Part model, mm, in its own coordinate system. A direction names the side the tool comes from. Round coordinates to 2 decimals unless told otherwise and drop trailing zeros. Write each loop counter-clockwise with the first axis right and the second up, starting at its lowest first coordinate (ties: lowest second). Pieces come first, ordered by that corner, then holes.
1) Flat gauge pins, fed straight in: pin 1 (9.5 mm diameter, centred on x = 35, y = 222, fed in from +Z); pin 2 (1 mm diameter, centred on x = -39, z = 9.5, fed in from -Y); pin 3 (6.5 mm diameter, centred on x = -8, z = 12.5, fed in from +Y); pin 4 (6 mm diameter, centred on y = 134.5, z = 13.5, fed in from +X). Where does each tip first touch, or does it go through?
2) Drill centre lines: L1, parallel to X at y = -141, z = 15.5; L2, parallel to Y at x = 35, z = 4; L3, parallel to Y at x = 132, z = 9.5. Where is each one in solid material? Low to high.
3) Pull direction Y, two halves, no side cores. Call faces 1 (the cylindrical face through (-186.88, -102.57, 8.11)), 2 (the flat face through (-224.978, 132.327, 12.056)), 3 (the flat face through (-227.09, -128.67, 12.06)): +Y half, -Y half, draft (parallel to the pull), parting line (faces both ways), or undercut.
4) Saw through at A-A on y = -111. Write the cut outline in (x, z).
5) Saw through at C-C on x = 101.5. Write the cut outline in (y, z), and give its area (3 significant figures).
6) Which spindle directions (+Z, -Z, +X, -X, +Y, -Y) get a long thin tool onto all of the face, cutting with end or side? Do faces 4 (the flat face through (224.978, -132.327, 12.056)), 5 (the flat face through (233.598, 137.397, 3.944)), 6 (the flat face through (227.09, 128.67, 12.06)), 7 (the flat face through (-1, 262, 8)). Say none if no direction does.
7) Saw through at B-B on z = 3. Count the separate pieces of the cut face and the enclosed holes in it, and give its area (3 significant figures).
8) Saw through at D-D on y = 68.5. Write the cut outline in (x, z), and give its area (3 significant figures).
```python
from build123d import *

# Parameters (mm, degrees)
BOSS_EXTRUDE1_DEPTH = 16
CUT_EXTRUDE1_REACH  = 426.953
SKETCH3_R           = 6
SKETCH4_OUTSIDE_W   = 813.904
SKETCH4_OUTSIDE_H   = 727.89
CUT_EXTRUDE2_DEPTH  = 8
SKETCH5_R           = 1.25
SKETCH5_R_2         = 10
CUT_EXTRUDE3_DEPTH  = 425.953330771
CUT_EXTRUDE6_DEPTH  = 425.953330771


with BuildPart() as part:
    # Sketch1 → Boss-Extrude1 (new body)
    with BuildSketch(Plane.XY):
        Polygon((160.503374835, 278), (-160.503374835, 278), (-321.006749669, 0), (-160.503374835, -278), (160.503374835, -278), (321.006749669, 0), align=None)
    extrude(amount=BOSS_EXTRUDE1_DEPTH)

    # Sketch3 → Cut-Extrude1 (cut, up to next)
    with BuildSketch(Plane.XY.offset(16), mode=Mode.PRIVATE) as cut_extrude1_sk1:
        with Locations((35, 222)):
            Circle(SKETCH3_R)
    cut_extrude1_tool1 = extrude(cut_extrude1_sk1.sketch, amount=-CUT_EXTRUDE1_REACH, mode=Mode.PRIVATE) & part.part
    # Sketch3 → Cut-Extrude1 (cut, up to next)
    with BuildSketch(Plane.XY.offset(16), mode=Mode.PRIVATE) as cut_extrude1_sk2:
        with Locations((-35, 222)):
            Circle(SKETCH3_R)
    cut_extrude1_tool2 = extrude(cut_extrude1_sk2.sketch, amount=-CUT_EXTRUDE1_REACH, mode=Mode.PRIVATE) & part.part
    # Sketch3 → Cut-Extrude1 (cut, up to next)
    with BuildSketch(Plane.XY.offset(16), mode=Mode.PRIVATE) as cut_extrude1_sk3:
        with Locations((-209.75763964, -80.689110868)):
            Circle(SKETCH3_R)
    cut_extrude1_tool3 = extrude(cut_extrude1_sk3.sketch, amount=-CUT_EXTRUDE1_REACH, mode=Mode.PRIVATE) & part.part
    # Sketch3 → Cut-Extrude1 (cut, up to next)
    with BuildSketch(Plane.XY.offset(16), mode=Mode.PRIVATE) as cut_extrude1_sk4:
        with Locations((-174.75763964, -141.310889132)):
            Circle(SKETCH3_R)
    cut_extrude1_tool4 = extrude(cut_extrude1_sk4.sketch, amount=-CUT_EXTRUDE1_REACH, mode=Mode.PRIVATE) & part.part
    # Sketch3 → Cut-Extrude1 (cut, up to next)
    with BuildSketch(Plane.XY.offset(16), mode=Mode.PRIVATE) as cut_extrude1_sk5:
        with Locations((174.75763964, -141.310889132)):
            Circle(SKETCH3_R)
    cut_extrude1_tool5 = extrude(cut_extrude1_sk5.sketch, amount=-CUT_EXTRUDE1_REACH, mode=Mode.PRIVATE) & part.part
    # Sketch3 → Cut-Extrude1 (cut, up to next)
    with BuildSketch(Plane.XY.offset(16), mode=Mode.PRIVATE) as cut_extrude1_sk6:
        with Locations((209.75763964, -80.689110868)):
            Circle(SKETCH3_R)
    cut_extrude1_tool6 = extrude(cut_extrude1_sk6.sketch, amount=-CUT_EXTRUDE1_REACH, mode=Mode.PRIVATE) & part.part
    add(cut_extrude1_tool1.solids().sort_by_distance((35, 222, 16))[0], mode=Mode.SUBTRACT)
    add(cut_extrude1_tool2.solids().sort_by_distance((-35, 222, 16))[0], mode=Mode.SUBTRACT)
    add(cut_extrude1_tool3.solids().sort_by_distance((-209.75764, -80.689111, 16))[0], mode=Mode.SUBTRACT)
    add(cut_extrude1_tool4.solids().sort_by_distance((-174.75764, -141.310889, 16))[0], mode=Mode.SUBTRACT)
    add(cut_extrude1_tool5.solids().sort_by_distance((174.75764, -141.310889, 16))[0], mode=Mode.SUBTRACT)
    add(cut_extrude1_tool6.solids().sort_by_distance((209.75764, -80.689111, 16))[0], mode=Mode.SUBTRACT)

    # Sketch4 outside → Cut-Extrude2 (cut)
    with BuildSketch(Plane.XY.offset(16)):
        Rectangle(SKETCH4_OUTSIDE_W, SKETCH4_OUTSIDE_H)
        Polygon((301.376840517, 0), (150.688420258, 261), (-150.688420258, 261), (-301.376840517, 0), (-150.688420258, -261), (150.688420258, -261), align=None, mode=Mode.SUBTRACT)
    extrude(amount=-CUT_EXTRUDE2_DEPTH, mode=Mode.SUBTRACT)

    # Sketch5 → Cut-Extrude3 (cut, through all)
    with BuildSketch(Plane.XY.offset(16)):
        with Locations((209.578147716, -121)):
            Circle(SKETCH5_R)
        with Locations((174.937131564, -101)):
            Circle(SKETCH5_R)
        with Locations((-192.25763964, -111)):
            Circle(SKETCH5_R_2)
        with Locations((0, 222)):
            Circle(SKETCH5_R_2)
        with Locations((-209.578147716, -121)):
            Circle(SKETCH5_R)
        with Locations((-174.937131564, -101)):
            Circle(SKETCH5_R)
        with Locations((0, 242)):
            Circle(SKETCH5_R)
        with Locations((0, 202)):
            Circle(SKETCH5_R)
        with Locations((192.25763964, -111)):
            Circle(SKETCH5_R_2)
    extrude(amount=-CUT_EXTRUDE3_DEPTH, mode=Mode.SUBTRACT)

    # Sketch8 → Cut-Extrude6 (cut, through all)
    with BuildSketch(Plane(origin=(0, 0, 0), x_dir=(-1, 0, 0), z_dir=(0, 0, -1))):
        Polygon((160.503374835, 278), (-160.503374835, 278), (-321.006749669, 0), (-160.503374835, -278), (160.503374835, -278), (321.006749669, 0), align=None)
        Polygon((156.46192295, 271), (-156.46192295, 271), (-312.923845901, 0), (-156.46192295, -271), (156.46192295, -271), (312.923845901, 0), align=None, mode=Mode.SUBTRACT)
    extrude(amount=-CUT_EXTRUDE6_DEPTH, mode=Mode.SUBTRACT)


solid = part.part
```
Completed:
1. pin 1: passes through
1. pin 2: stops at y = -261
1. pin 3: stops at y = 261
1. pin 4: stops at x = 225.46
2. L1: x = -219.97 to -180.75, -168.77 to 168.77, 180.75 to 219.97
2. L2: y = -271 to 216, 228 to 271
2. L3: y = -261 to 261
3. face 1: undercut
3. face 2: +Y half
3. face 3: -Y half
4. outline: (-248.84, 0) - (-202.26, 0) - (-202.26, 16) - (-237.29, 16) - (-237.29, 8) - (-248.84, 8) - close; (-182.26, 0) - (182.26, 0) - (182.26, 16) - (-182.26, 16) - close; (202.26, 0) - (248.84, 0) - (248.84, 8) - (237.29, 8) - (237.29, 16) - (202.26, 16) - close
5. outline: (-271, 0) - (271, 0) - (271, 8) - (261, 8) - (261, 16) - (-261, 16) - (-261, 8) - (-271, 8) - close
5. area: 8,510 mm2
6. face 4: +Z, +X, -Y
6. face 5: +Z, -Z, +X, +Y
6. face 6: +Z, +X, +Y
6. face 7: +Z
7. separate pieces: 1
7. enclosed holes: 15
7. area: 253,000 mm2
8. outline: (-273.38, 0) - (273.38, 0) - (273.38, 8) - (261.83, 8) - (261.83, 16) - (-261.83, 16) - (-261.83, 8) - (-273.38, 8) - close
8. area: 8,560 mm2
